```python
from build123d import *

# Parameters (mm, degrees)
EXTRUDE_1_DEPTH = 5
FILLET_1_R      = 2


with BuildPart() as part:
    # 草图1 → 凸台-拉伸1 (new body)
    with BuildSketch(Plane.XY):
        Polygon((-30, 24), (30, 24), (30, -24), (9.2, -24), (9.2, 16), (-9.2, 16), (-9.2, -24), (-30, -24), align=None)
    extrude(amount=EXTRUDE_1_DEPTH)

    # 圆角1
    fillet_1_edges = [part.edges().sort_by_distance(p)[0] for p in [
        (9.2, -24, 2.5),
        (-9.2, -24, 2.5),
        (-30, -24, 2.5),
        (-30, 24, 2.5),
        (30, 24, 2.5),
        (30, -24, 2.5),
    ]]
    fillet(fillet_1_edges, radius=FILLET_1_R)


solid = part.part
```
The model under review builds one solid part; all positions refer to its coordinate system, in mm. A direction names the side the tool comes from. Give positions to 0.01 mm unless a question says otherwise; leave off trailing zeros. Write each loop counter-clockwise with the first axis right and the second up, starting at its lowest first coordinate (ties: lowest second). Pieces come first, ordered by that corner, then holes.
(1) The part is to be moulded in two halves that separate along X. For faces 3 (the flat face through (14, 0, 0)), 4 (the flat face through (30, 0, 2)), 5 (the flat face through (9.2, -3, 2)), say which applies: released by +X, released by -X, zero draft, split by the parting line, or undercut.
(2) Tool access review of faces 1 (the cylindrical face through (-29.4, 23.43, 2.54)), 2 (the cylindrical face through (-9.77, -23.4, 2.54)): name each direction out of +Z, -Z, +X, -X, +Y, -Y from which nothing blocks a thin tool from reaching the whole face with its end or side.
(3) Consider section A-A, the plane y = -5. Give the boundary of the cut face in (x, z), and give its area (3 significant figures).
(4) To check wall thickness, follow L1, parallel to X at y = 9, z = 0.7; L2, parallel to Y at x = -9, z = 0.8. State the ranges of each line that lie inside material, in increasing order.
(5) For P1, Ø2.5, axis at x = -2, z = 2, coming from the -Y side; P2, Ø10, axis at x = -6, y = 13.5, coming from the +Z side; P3, Ø4, axis at x = 5.5, y = -10, coming from the +Z side, all flat-tipped, find the tip position at first contact; note any pin that passes through.
(6) Consider section B-B, the plane z = 0.75. Give the boundary of the cut face in (x, y), and give its area (3 significant figures).
(7) Consider section C-C, the plane x = 4.5. Give the boundary of the cut face in (y, z).
Returned:
1. face 3: zero draft
1. face 4: released by +X
1. face 5: undercut
2. face 1: +Z, -Z, -X, +Y
2. face 2: +Z, -Z, -Y
3. outline: (-30, 0) - (-9.2, 0) - (-9.2, 5) - (-30, 5) - close; (9.2, 0) - (30, 0) - (30, 5) - (9.2, 5) - close
3. area: 208 mm2
4. L1: x = -30 to -9.2, 9.2 to 30
4. L2: y = 16 to 24
5. P1: stops at y = 16
5. P2: stops at z = 5
5. P3: passes through
6. outline: (-30, -22) arc R2 ccw to (-28, -24) - (-11.2, -24) arc R2 ccw to (-9.2, -22) - (-9.2, 16) - (9.2, 16) - (9.2, -22) arc R2 ccw to (11.2, -24) - (28, -24) arc R2 ccw to (30, -22) - (30, 22) arc R2 ccw to (28, 24) - (-28, 24) arc R2 ccw to (-30, 22) - close
6. area: 2,140 mm2
7. outline: (16, 0) - (24, 0) - (24, 5) - (16, 5) - close
